Work out the finished part from the listing and answer in its coordinate system (mm). Face numbers are marked on the shaded views. A direction names the side the tool comes from. Round coordinates to 2 decimals unless told otherwise and drop trailing zeros. Order: outer loops, then holes, each group sorted by start corner. A loop starts at its lowest first (then second) coordinate and runs counter-clockwise, first axis right, second up. Notation, with made-up numbers: (-37, 45.5) - (-13, 45.5) arc R14 ccw to (-13, 49.5) - close; hole circle Ø3 at (84, 41.25). An arc over 180 degrees is marked (long way). Answer in a Markdown table with one row per item.
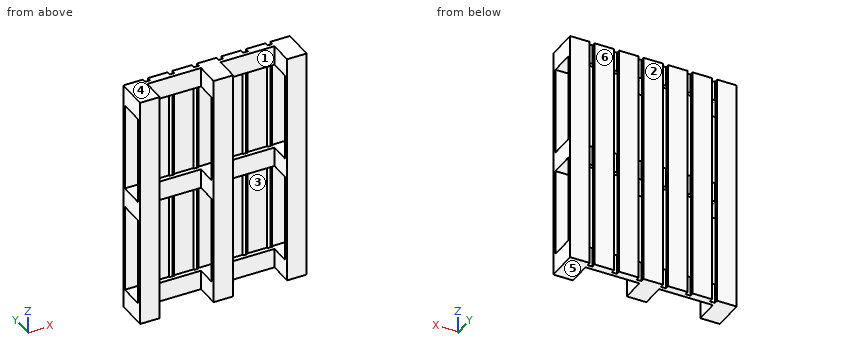
from build123d import *

# Parameters (mm, degrees)
SKETCH1_W           = 850
SKETCH1_H           = 160
BOSS_EXTRUDE1_DEPTH = 1200
SKETCH2_W           = 275
SKETCH2_H           = 120
CUT_EXTRUDE1_DEPTH  = 1480.222768889
SKETCH3_W           = 450
SKETCH3_H           = 125
CUT_EXTRUDE2_DEPTH  = 1480.222768889
SKETCH4_W           = 25
SKETCH4_H           = 20
CUT_EXTRUDE3_DEPTH  = 1480.222768889


with BuildPart() as part:
    # Sketch1 → Boss-Extrude1 (new body)
    with BuildSketch(Plane.XY):
        with Locations((425, 80)):
            Rectangle(SKETCH1_W, SKETCH1_H)
    extrude(amount=-BOSS_EXTRUDE1_DEPTH)

    # Sketch2 → Cut-Extrude1 (cut, through all)
    with BuildSketch(Plane.XY):
        with Locations((237.5, 60)):
            Rectangle(SKETCH2_W, SKETCH2_H)
        with Locations((612.5, 60)):
            Rectangle(SKETCH2_W, SKETCH2_H)
    extrude(amount=-CUT_EXTRUDE1_DEPTH, mode=Mode.SUBTRACT)

    # Sketch3 → Cut-Extrude2 (cut, through all)
    with BuildSketch(Plane.ZY):
        with Locations((-875, 82.5)):
            Rectangle(SKETCH3_W, SKETCH3_H)
        with Locations((-325, 82.5)):
            Rectangle(SKETCH3_W, SKETCH3_H)
    extrude(amount=-CUT_EXTRUDE2_DEPTH, mode=Mode.SUBTRACT)

    # Sketch4 → Cut-Extrude3 (cut, through all)
    with BuildSketch(Plane.XY):
        with Locations((112.5, 150)):
            Rectangle(SKETCH4_W, SKETCH4_H)
        with Locations((237.5, 150)):
            Rectangle(SKETCH4_W, SKETCH4_H)
        with Locations((362.5, 150)):
            Rectangle(SKETCH4_W, SKETCH4_H)
        with Locations((487.5, 150)):
            Rectangle(SKETCH4_W, SKETCH4_H)
        with Locations((612.5, 150)):
            Rectangle(SKETCH4_W, SKETCH4_H)
        with Locations((737.5, 150)):
            Rectangle(SKETCH4_W, SKETCH4_H)
    extrude(amount=-CUT_EXTRUDE3_DEPTH, mode=Mode.SUBTRACT)


solid = part.part
1) The mould has two halves that part along Z. Classify the marked faces 3, 4, 5 and 6: released by +Z, released by -Z, zero draft, split by the parting line, or undercut.
Filled in:
| item | result |
|---|---|
| face 3 | undercut |
| face 4 | released by +Z |
| face 5 | released by -Z |
| face 6 | zero draft |
2) This flat-tipped pin is pushed along its axis until it touches: pin 1 (7.5 mm diameter, centred on x = 615, z = -70, fed in from +Y). Where does it stop, or does it pass through?
Filled in:
| item | result |
|---|---|
| pin 1 | stops at y = 140 |
3) Find section A-A, the plane x = 798.5. Give the vertices of the cut face in (y, z), then the cut area to 3 significant figures.
Filled in:
| item | result |
|---|---|
| outline | (0, -1200) - (160, -1200) - (160, 0) - (0, 0) - close; hole (20, -1100) - (145, -1100) - (145, -650) - (20, -650) - close; hole (20, -550) - (145, -550) - (145, -100) - (20, -100) - close |
| area | 79,500 mm^2 |
4) Find section D-D, the plane x = 640. Give the vertices of the cut face in (y, z).
Filled in:
| item | result |
|---|---|
| outline | (120, -1200) - (160, -1200) - (160, 0) - (120, 0) - (120, -100) - (145, -100) - (145, -550) - (120, -550) - (120, -650) - (145, -650) - (145, -1100) - (120, -1100) - close |
5) Find the intervals of material crossed by probe 1 along Z at (x, y) = (425, 85); probe 2 along Y at (x, z) = (41, -121.5); probe 3 along X at (y, z) = (46, -1142.5), in increasing order. Write a range as from..to.
Filled in:
| item | result |
|---|---|
| probe 1 | z = -1200..-1100, -650..-550, -100..0 |
| probe 2 | y = 0..20, 145..160 |
| probe 3 | x = 0..100, 375..475, 750..850 |
6) Which of the six approach directions +Z, -Z, +X, -X, +Y, -Y give full straight-line access (tool end or side, diameter ignored) to the marked faces 1 and 2?
Filled in:
| item | result |
|---|---|
| face 1 | +Z, -Z, -Y |
| face 2 | +Z, -Z, +X, -X, +Y |
7) Find section B-B, the plane z = -871. Give the number of separate pieces and of enclosed holes in the cut face, then the cut area to 3 significant figures.
Filled in:
| item | result |
|---|---|
| separate pieces | 10 |
| enclosed holes | 0 |
| area | 16,500 mm^2 |
